Geometry check sheet. Reference: the model listing, model coordinates, mm. A direction names the side the tool comes from. Coordinates: 2 decimals unless noted, no trailing zeros. Write each loop counter-clockwise with the first axis right and the second up, starting at its lowest first coordinate (ties: lowest second). Pieces come first, ordered by that corner, then holes. Notation, with made-up numbers: (-1.5, 24) -> (40.5, 24) arc R21 ccw to (40.5, 42) -> close; hole circle Ø11 at (12.5, -6.5). An arc over 180 degrees is marked (long way). Answer in a Markdown table with one row per item. Add a question column.
Q1. Section check C-C, the plane z = 18.5. Record the boundary of the cut face in (x, y), and give its area (3 significant figures).
Q2. Section check D-D, the plane x = -17. Record the boundary of the cut face in (y, z).
Q3. Section check B-B, the plane x = 30. Record the boundary of the cut face in (y, z), and give its area (3 significant figures).
Q4. Tool access check on faces 1 (the face through (-40, -17, 18)), 2 (the face through (-38, -16, 18)). Record the directions out of +Z, -Z, +X, -X, +Y, -Y that give a thin tool (end or side, any length) a straight path to the whole face; none if there is none.
Q5. Gauge pin test, flat ends, axial feed: P1, Ø4, axis at x = -8.5, z = 17, coming from the +Y side; P2, Ø0.6, axis at y = -18.5, z = 31, coming from the -X side; P3, Ø2, axis at y = -15, z = 4, coming from the +X side. Record the tip position at first contact, or that the pin passes through.
Q6. Section check A-A, the plane y = -17. Record the boundary of the cut face in (x, z).
Q7. Release check for a two-part mould opening along Z. For faces 3 (the face through (-39.008, -15.897, 30.755)), 4 (the face through (31.66, -18.99, 6.13)), 5 (the face through (-39, -14, 18)) record: pulls with the +Z half, pulls with the -Z half, needs draft (parallel to the pull), parting line crosses it, or undercut.
Q8. Thickness scan on line 1 (Z direction, x = -38.85, y = -17); line 2 (Z direction, x = 30, y = -18.65); line 3 (X direction, y = -18.65, z = 6.5). Record the ranges inside material, lowest first.
```python
from build123d import *

# Parameters (mm, degrees)
SKETCH_1_W                  = 80
SKETCH_1_H                  = 40
SKETCH_1_W_2                = 76
SKETCH_1_H_2                = 36
EXTRUDE_1_DEPTH             = 36
CUT_EXTRUDE_1_DEPTH         = 37
HOLE_WIZARD_4_40_AT_2_COUNT = 2
HOLE_WIZARD_4_40_AT_2_PITCH = 26
HOLE_WIZARD_M3_AT_2_COUNT   = 2
HOLE_WIZARD_M3_AT_2_PITCH   = 23


with BuildPart() as part:
    # Эскиз1 → Бобышка-Вытянуть1 (new body)
    with BuildSketch(Plane.XY):
        Rectangle(SKETCH_1_W, SKETCH_1_H)
        Rectangle(SKETCH_1_W_2, SKETCH_1_H_2, mode=Mode.SUBTRACT)
    extrude(amount=EXTRUDE_1_DEPTH)

    # Эскиз2 → Вырез-Вытянуть1 (cut, through all)
    with BuildSketch(Plane.XY.offset(36)):
        Polygon((-40, 20), (-40, -14), (-38, -14), (-38, 18), (38, 18), (38, -18), (36, -18), (36, -20), (40, -20), (40, 20), align=None)
    extrude(amount=-CUT_EXTRUDE_1_DEPTH, mode=Mode.SUBTRACT)

    # Эскиз3 → 4-40 (revolve, cut)
    with BuildSketch(Plane(origin=(-40, -17, 5), x_dir=(0, 0, 1), z_dir=(0, 1, 0))):
        Polygon((0, 0), (0, 2), (1.524, 2), (1.1303, 1.6063), (1.1303, 0.3937), (1.524, 0), align=None)
    hole_wizard_4_40 = revolve(axis=Axis((-46.35, -17, 5), (1, 0, 0)), mode=Mode.SUBTRACT)

    # 4-40 at 2: 4-40 ×2
    with Locations(*[(0, 0, i * HOLE_WIZARD_4_40_AT_2_PITCH) for i in range(1, HOLE_WIZARD_4_40_AT_2_COUNT)]):
        add(hole_wizard_4_40, mode=Mode.SUBTRACT)

    # Эскиз5 → Отверстие под  M3 (revolve, cut)
    with BuildSketch(Plane(origin=(30, -18, 6.5), x_dir=(0, 0, 1), z_dir=(1, 0, 0))):
        Polygon((0, 0), (0, 2), (1.8, 2), (1.7, 1.9), (1.7, 0.1), (1.8, 0), align=None)
    hole_wizard_m3 = revolve(axis=Axis((30, -11.65, 6.5), (0, -1, 0)), mode=Mode.SUBTRACT)

    # Отверстие под  M3 at 2: Отверстие под  M3 ×2
    with Locations(*[(0, 0, i * HOLE_WIZARD_M3_AT_2_PITCH) for i in range(1, HOLE_WIZARD_M3_AT_2_COUNT)]):
        add(hole_wizard_m3, mode=Mode.SUBTRACT)


solid = part.part
```
Calculated:
| question | item | result |
|---|---|---|
| 1 | outline | (-40, -20) -> (36, -20) -> (36, -18) -> (-38, -18) -> (-38, -14) -> (-40, -14) -> close |
| 1 | area | 160 mm² |
| 2 | outline | (-20, 0) -> (-18, 0) -> (-18, 36) -> (-20, 36) -> close |
| 3 | outline | (-20, 0) -> (-18, 0) -> (-18, 4.7) -> (-18.1, 4.8) -> (-19.9, 4.8) -> (-20, 4.7) -> close; (-20, 8.3) -> (-19.9, 8.2) -> (-18.1, 8.2) -> (-18, 8.3) -> (-18, 27.7) -> (-18.1, 27.8) -> (-19.9, 27.8) -> (-20, 27.7) -> close; (-20, 31.3) -> (-19.9, 31.2) -> (-18.1, 31.2) -> (-18, 31.3) -> (-18, 36) -> (-20, 36) -> close |
| 3 | area | 58.4 mm² |
| 4 | face 1 | +Z, -Z, -X, +Y, -Y |
| 4 | face 2 | +Z, -Z, +X, +Y |
| 5 | P1 | stops at y = -18 |
| 5 | P2 | stops at x = -40 |
| 5 | P3 | stops at x = -38 |
| 6 | outline | (-40, 0) -> (-38, 0) -> (-38, 3.48) -> (-38.39, 3.87) -> (-39.61, 3.87) -> (-40, 3.48) -> close; (-40, 6.52) -> (-39.61, 6.13) -> (-38.39, 6.13) -> (-38, 6.52) -> (-38, 29.48) -> (-38.39, 29.87) -> (-39.61, 29.87) -> (-40, 29.48) -> close; (-40, 32.52) -> (-39.61, 32.13) -> (-38.39, 32.13) -> (-38, 32.52) -> (-38, 36) -> (-40, 36) -> close |
| 7 | face 3 | undercut |
| 7 | face 4 | undercut |
| 7 | face 5 | needs draft |
| 8 | line 1 | z = 0 to 3.87, 6.13 to 29.87, 32.13 to 36 |
| 8 | line 2 | z = 0 to 4.8, 8.2 to 27.8, 31.2 to 36 |
| 8 | line 3 | x = -40 to 28.3, 31.7 to 36 |
